```python
from build123d import *

# Parameters (mm, degrees)
F0_W     = 20
F0_H     = 25
F0_R     = 7.3
F1_DEPTH = 30
F4_DEPTH = 25.001
F5_W     = 20
F5_H     = 25
F6_DEPTH = 2


with BuildPart() as f1:
    # F0 (on Top) → F1 (new body)
    with BuildSketch(Plane.XY):
        Rectangle(F0_W, F0_H)
        Circle(F0_R, mode=Mode.SUBTRACT)
    extrude(amount=F1_DEPTH)

    # F3 (on face) → F4 (cut, through all)
    with BuildSketch(Plane(origin=(0, 12.5, 0), x_dir=(-1, 0, 0), z_dir=(0, 1, 0))):
        with BuildLine():
            ThreePointArc((0, 5.85), (-1.6, 4.25), (0, 2.65))
            Line((0, 2.65), (0, 4.25))
            Line((0, 4.25), (0, 5.85))
        make_face()
        with BuildLine():
            ThreePointArc((1.6, 23.25), (-1.1313708499, 24.3813708499), (0, 21.65))
            ThreePointArc((0, 21.65), (1.1313708499, 22.1186291501), (1.6, 23.25))
        make_face()
        with BuildLine():
            ThreePointArc((0, 17.75), (-4, 13.75), (0, 9.75))
            Line((0, 9.75), (0, 17.75))
        make_face()
        with BuildLine():
            Line((0, 17.75), (0, 9.75))
            ThreePointArc((0, 9.75), (2.8284271247, 10.9215728753), (4, 13.75))
            ThreePointArc((4, 13.75), (2.8284271247, 16.5784271247), (0, 17.75))
        make_face()
        with BuildLine():
            Line((0, 4.25), (0, 2.65))
            ThreePointArc((0, 2.65), (1.1313708499, 3.1186291501), (1.6, 4.25))
            ThreePointArc((1.6, 4.25), (1.1313708499, 5.3813708499), (0, 5.85))
            Line((0, 5.85), (0, 4.25))
        make_face()
    extrude(amount=-F4_DEPTH, mode=Mode.SUBTRACT)

    # F5 (on face) → F6 (join)
    with BuildSketch(Plane(origin=(0, 0, 0), x_dir=(1, 0, 0), z_dir=(0, 0, -1))):
        Rectangle(F5_W, F5_H)
    extrude(amount=F6_DEPTH)


solid = f1.part
```
Could you check a few things on this model? Use its own coordinates, in mm. A direction names the side the tool comes from. Round coordinates to 2 decimals unless told otherwise and drop trailing zeros. Write each loop counter-clockwise with the first axis right and the second up, starting at its lowest first coordinate (ties: lowest second). Pieces come first, ordered by that corner, then holes. Notation, with made-up numbers: M 28,74 L 65,74 A11 ccw 65,87 Z; hole C 51.25,30.25 d10. An arc over 180 degrees is marked long. Answer in a Markdown table with one row per item. Add a question column.
Q1. On a 3-axis mill with a long thin cutter (end or side, diameter ignored), from which of +Z, -Z, +X, -X, +Y, -Y can I reach the whole of each face in a straight line? I mean faces 1 (the flat face through (10, 0, 14)), 2 (the cylindrical face through (6.74, -2.8, 14.79)). Say none if no direction works.
Q2. Imagine slicing it at D-D (z = 8). Please give me the cut outline in (x, y), then the cut area to 3 significant figures.
Q3. Will these pins go through, and if not, where does the flat tip stop? pin 1 Ø11.5 at (x, y) = (0, 0) entering from +Z; pin 2 Ø8 at (x, y) = (4, -1) entering from +Z.
Q4. Imagine slicing it at B-B (y = 9.5). Please give me the cut outline in (x, z).
Q5. If I drill on line 1 (Y direction, x = -4, z = 6); line 2 (X direction, y = -9.65, z = 23.25); line 3 (Z direction, x = 5.25, y = 1.5), over which ranges is the centre line in solid material (lowest first)? Write a range as from..to.
Q6. Imagine slicing it at A-A (z = 15). Please give me the cut outline in (x, y), then the cut area to 3 significant figures.
Q7. Imagine slicing it at C-C (y = 0). Please give me the cut outline in (x, z).
Values:
| question | item | result |
|---|---|---|
| 1 | face 1 | +Z, -Z, +X, +Y, -Y |
| 1 | face 2 | +Z |
| 2 | outline | M -10,-12.5 L 10,-12.5 L 10,12.5 L -10,12.5 Z; hole C 0,0 d14.6 |
| 2 | area | 333 mm^2 |
| 3 | pin 1 | z = 0 |
| 3 | pin 2 | z = 30 |
| 4 | outline | M -10,-2 L 10,-2 L 10,30 L -10,30 Z; hole C 0,13.75 d8; hole C 0,4.25 d3.2; hole C 0,23.25 d3.2 |
| 5 | line 1 | -12.5..-6.11, 6.11..12.5 |
| 5 | line 2 | -10..-1.6, 1.6..10 |
| 5 | line 3 | -2..0 |
| 6 | outline | M -10,-12.5 L -3.8,-12.5 L -3.8,-6.23 A7.3 cw -3.8,6.23 L -3.8,12.5 L -10,12.5 Z; M 3.8,-12.5 L 10,-12.5 L 10,12.5 L 3.8,12.5 L 3.8,6.23 A7.3 cw 3.8,-6.23 Z |
| 6 | area | 248 mm^2 |
| 7 | outline | M -10,-2 L 10,-2 L 10,30 L 7.3,30 L 7.3,0 L -7.3,0 L -7.3,30 L -10,30 Z |
